```python
from build123d import *

# Parameters (mm, degrees)
SKETCH_1_R           = 21
EXTRUDE_2_DEPTH      = 26.4
SKETCH_10_R          = 18.4
CUT_EXTRUDE_5_DEPTH  = 24
SKETCH_11_R          = 1.5
CUT_EXTRUDE_6_DEPTH  = 24
EXTRUDE_START        = 4
SKETCH_13_R          = 24.5
SKETCH_13_R_2        = 21
EXTRUDE_4_DEPTH      = 4
SKETCH_14_R          = 1.5
CUT_EXTRUDE_7_DEPTH  = 4
SKETCH_16_R          = 21
SKETCH_16_R_2        = 19
CUT_EXTRUDE_10_DEPTH = 1
SKETCH_27_R          = 21
SKETCH_27_R_2        = 20
CUT_EXTRUDE_14_DEPTH = 20
SKETCH_29_R          = 20
SKETCH_29_R_2        = 19
CUT_EXTRUDE_15_DEPTH = 1
CUT_EXTRUDE_16_DEPTH = 10
SKETCH_32_R          = 26
SKETCH_32_R_2        = 24.5
EXTRUDE_5_DEPTH      = 4


with BuildPart() as part:
    # 草图1 → 凸台-拉伸2 (new body)
    with BuildSketch(Plane(origin=(0, 0, 0), x_dir=(1, 0, 0), z_dir=(0, 1, 0))):
        with Locations(Location((0, 0, 0), (0, 0, 270))):
            Circle(SKETCH_1_R)
    extrude(amount=EXTRUDE_2_DEPTH)

    # 草图10 → 切除-拉伸5 (cut)
    with BuildSketch(Plane(origin=(0, 26.4, 0), x_dir=(1, 0, 0), z_dir=(0, 1, 0))):
        with Locations(Location((0, 0, 0), (0, 0, 270))):
            Circle(SKETCH_10_R)
    extrude(amount=-CUT_EXTRUDE_5_DEPTH, mode=Mode.SUBTRACT)

    # 草图11 → 切除-拉伸6 (cut)
    with BuildSketch(Plane.XZ):
        with Locations(Location((-0.993017559, 15.468158136, 0), (0, 0, 270))):
            Circle(SKETCH_11_R)
        with Locations(Location((12.899309116, 8.594057501, 0), (0, 0, 270))):
            Circle(SKETCH_11_R)
        with Locations(Location((13.892326675, -6.874100635, 0), (0, 0, 270))):
            Circle(SKETCH_11_R)
        with Locations(Location((0.993017559, -15.468158136, 0), (0, 0, 270))):
            Circle(SKETCH_11_R)
        with Locations(Location((-12.899309116, -8.594057501, 0), (0, 0, 270))):
            Circle(SKETCH_11_R)
        with Locations(Location((-13.892326675, 6.874100635, 0), (0, 0, 270))):
            Circle(SKETCH_11_R)
    extrude(amount=-CUT_EXTRUDE_6_DEPTH, mode=Mode.SUBTRACT)

    # 草图13 → 凸台-拉伸4 (add)
    with BuildSketch(Plane(origin=(0, 4, 0), x_dir=(-1, 0, 0), z_dir=(0, -1, 0)).offset(EXTRUDE_START)):
        with Locations(Location((0, 0, 0), (0, 0, 90))):
            Circle(SKETCH_13_R)
        with Locations(Location((0, 0, 0), (0, 0, 90))):
            Circle(SKETCH_13_R_2, mode=Mode.SUBTRACT)
    extrude(amount=-EXTRUDE_4_DEPTH)

    # 草图14 → 切除-拉伸7 (cut)
    with BuildSketch(Plane(origin=(0, 4, 0), x_dir=(1, 0, 0), z_dir=(0, 1, 0))):
        with Locations(Location((1.457493515, 22.703264361, 0), (0, 0, 270))):
            Circle(SKETCH_14_R)
        with Locations(Location((22.703264361, -1.457493515, 0), (0, 0, 270))):
            Circle(SKETCH_14_R)
        with Locations(Location((-1.457493515, -22.703264361, 0), (0, 0, 270))):
            Circle(SKETCH_14_R)
        with Locations(Location((-22.703264361, 1.457493515, 0), (0, 0, 270))):
            Circle(SKETCH_14_R)
    extrude(amount=-CUT_EXTRUDE_7_DEPTH, mode=Mode.SUBTRACT)

    # 草图16 → 切除-拉伸10 (cut)
    with BuildSketch(Plane(origin=(0, 13, 0), x_dir=(-1, 0, 0), z_dir=(0, -1, 0))):
        with Locations(Location((0, 0, 0), (0, 0, 90))):
            Circle(SKETCH_16_R)
        with Locations(Location((0, 0, 0), (0, 0, 90))):
            Circle(SKETCH_16_R_2, mode=Mode.SUBTRACT)
    extrude(amount=-CUT_EXTRUDE_10_DEPTH, mode=Mode.SUBTRACT)

    # 草图27 → 切除-拉伸14 (cut)
    with BuildSketch(Plane.XZ.offset(-14)):
        with Locations(Location((0, 0, 0), (0, 0, 270))):
            Circle(SKETCH_27_R)
        with Locations(Location((0, 0, 0), (0, 0, 270))):
            Circle(SKETCH_27_R_2, mode=Mode.SUBTRACT)
    extrude(amount=-CUT_EXTRUDE_14_DEPTH, mode=Mode.SUBTRACT)

    # 草图29 → 切除-拉伸15 (cut)
    with BuildSketch(Plane(origin=(0, 23, 0), x_dir=(-1, 0, 0), z_dir=(0, -1, 0))):
        with Locations(Location((0, 0, 0), (0, 0, 90))):
            Circle(SKETCH_29_R)
        with Locations(Location((0, 0, 0), (0, 0, 90))):
            Circle(SKETCH_29_R_2, mode=Mode.SUBTRACT)
    extrude(amount=-CUT_EXTRUDE_15_DEPTH, mode=Mode.SUBTRACT)

    # 草图31 → 切除-拉伸16 (cut)
    with BuildSketch(Plane.XZ):
        with BuildLine():
            Line((7, -6.018809273), (-6.401397723, -6.018809273))
            ThreePointArc((-6.401397723, -6.018809273), (-12.420206996, 0), (-6.401397723, 6.018809273))
            Line((-6.401397723, 6.018809273), (7, 6.018809273))
            ThreePointArc((7, 6.018809273), (13.018809273, 0), (7, -6.018809273))
        make_face()
    extrude(amount=-CUT_EXTRUDE_16_DEPTH, mode=Mode.SUBTRACT)

    # 草图32 → 凸台-拉伸5 (add)
    with BuildSketch(Plane.XZ):
        with Locations(Location((0, 0, 0), (0, 0, 270))):
            Circle(SKETCH_32_R)
        Circle(SKETCH_32_R_2, mode=Mode.SUBTRACT)
    extrude(amount=-EXTRUDE_5_DEPTH)


solid = part.part
```
Part model, mm, in its own coordinate system. A direction names the side the tool comes from. Round coordinates to 2 decimals unless told otherwise and drop trailing zeros. Order: outer loops, then holes, each group sorted by start corner. A loop starts at its lowest first (then second) coordinate and runs counter-clockwise, first axis right, second up. Notation, with made-up numbers: M 32,34 L 58,34 A13 cw 58,41 Z; hole C 6,-6.75 d2. An arc over 180 degrees is marked long. Answer in a Markdown table with one row per item. Add a question column.
Q1. 3-axis set-ups, long thin cutter, end or side, ignore diameter. For faces 1 (the face through (-11, 13, 16)), 2 (the face through (0, 1, -6.019)), 3 (the face through (-19.524, 18.437, 4.336)): which of +Z, -Z, +X, -X, +Y, -Y reach the whole face in a straight line?
Q2. Cut at C-C on z = -13. Give the cut face in (x, y), and give its area (3 significant figures).
Q3. Wall check: L1, parallel to Y at x = 13, z = -14.5; L2, parallel to X at y = 10.25, z = 0; L3, parallel to X at y = 1.5, z = -2. Give the ranges that are in metal, low to high. Write a range as from..to.
Q4. Mould opens along X. For faces 4 (the face through (2, 4, -21.1)), 5 (the face through (-11.56, 13.49, 15.08)), 6 (the face through (-1.392, 2.028, 21.205)) say: +X half, -X half, draft (parallel to the pull), parting line (faces both ways), or undercut.
Q5. Cut at A-A on y = 10.25. Give the cut face in (x, z).
Q6. Pin check, flat tips, straight feed: pin 1 (5 mm diameter, centred on x = -13.89, z = 6.87, fed in from -Y); pin 2 (4 mm diameter, centred on x = -12, y = 14, fed in from +Z); pin 3 (6 mm diameter, centred on y = 9, z = -12, fed in from -X); pin 4 (2 mm diameter, centred on x = -19, z = 16, fed in from +Y). Stop position of each tip, or through.
Q7. Cut at D-D on y = 1.75. Give the number of separate pieces and of enclosed holes in the cut face, and give its area (3 significant figures).
Established:
| question | item | result |
|---|---|---|
| 1 | face 1 | none |
| 1 | face 2 | +Y, -Y |
| 1 | face 3 | +Y |
| 2 | outline | M -22.52,0 L 22.52,0 L 22.52,4 L 16.49,4 L 16.49,13 L 13.86,13 L 13.86,14 L 15.2,14 L 15.2,23 L 13.86,23 L 13.86,24 L 15.2,24 L 15.2,26.4 L 13.02,26.4 L 13.02,2.4 L -13.02,2.4 L -13.02,26.4 L -15.2,26.4 L -15.2,24 L -13.86,24 L -13.86,23 L -15.2,23 L -15.2,14 L -13.86,14 L -13.86,13 L -16.49,13 L -16.49,4 L -22.52,4 Z |
| 2 | area | 254 mm2 |
| 3 | L1 | y = 0..13, 14..23, 24..26.4 |
| 3 | L2 | x = -21..-18.4, 18.4..21 |
| 3 | L3 | x = -25.92..-24.1, -21.3..-12.08, 12.68..25.92 |
| 4 | face 4 | draft |
| 4 | face 5 | parting line |
| 4 | face 6 | undercut |
| 5 | outline | C 0,0 d42; hole C 0,0 d36.8 |
| 6 | pin 1 | stops at y = 0 |
| 6 | pin 2 | stops at z = 18.32 |
| 6 | pin 3 | stops at x = -18.97 |
| 6 | pin 4 | stops at y = 4 |
| 7 | separate pieces | 1 |
| 7 | enclosed holes | 11 |
| 7 | area | 1,780 mm2 |
